```python
from build123d import *

# Parameters (mm, degrees)
SKETCH1_W           = 42
SKETCH1_H           = 62
SKETCH1_R           = 4.15
BOSS_EXTRUDE1_DEPTH = 10
FILLET1_R           = 3
SKETCH2_R           = 2.6
CUT_EXTRUDE1_DEPTH  = 11
SKETCH3_R           = 9.45
CUT_EXTRUDE2_DEPTH  = 10


with BuildPart() as part:
    # Sketch1 → Boss-Extrude1 (new body)
    with BuildSketch(Plane.XY):
        with Locations((21, 31)):
            Rectangle(SKETCH1_W, SKETCH1_H)
        with Locations((21, 42)):
            Circle(SKETCH1_R, mode=Mode.SUBTRACT)
    extrude(amount=BOSS_EXTRUDE1_DEPTH)

    # Fillet1
    fillet1_edges = [part.edges().sort_by_distance(p)[0] for p in [
        (0, 62, 5),
        (42, 62, 5),
    ]]
    fillet(fillet1_edges, radius=FILLET1_R)

    # Sketch2 → Cut-Extrude1 (cut, through all)
    with BuildSketch(Plane.XY.offset(10)):
        with Locations((5, 7.5)):
            Circle(SKETCH2_R)
        with Locations((21, 7.5)):
            Circle(SKETCH2_R)
        with Locations((37, 7.5)):
            Circle(SKETCH2_R)
    extrude(amount=-CUT_EXTRUDE1_DEPTH, mode=Mode.SUBTRACT)

    # Sketch3 → Cut-Extrude2 (cut)
    with BuildSketch(Plane.XY.offset(10)):
        with Locations((21, 42)):
            Circle(SKETCH3_R)
    extrude(amount=-CUT_EXTRUDE2_DEPTH, mode=Mode.SUBTRACT)


solid = part.part
```
Source: CAD feature listing. Evaluate the final solid. Frame: model axes, mm. Round coordinates to 2 decimals unless told otherwise and drop trailing zeros. Loops run counter-clockwise (first coordinate to the right, second up) from the corner with the lowest first, then second, coordinate; pieces in that order, holes last. Notation, with made-up numbers: M 43,66.5 L 53,66.5 A22 cw 53,97.5 Z; hole C -15.75,-28.5 d4. An arc over 180 degrees is marked long. Put each result on its own line as item: value.
(1) Section C-C, the plane x = 21. Return loops of the section in (y, z), and give its area (3 significant figures).
Solutions:
outline: M 0,0 L 4.9,0 L 4.9,10 L 0,10 Z; M 10.1,0 L 32.55,0 L 32.55,10 L 10.1,10 Z; M 51.45,0 L 62,0 L 62,10 L 51.45,10 Z
area: 379 mm²
(2) Ray query, line 1 (Y direction, x = 5, z = 7); line 2 (Y direction, x = 13, z = 7); line 3 (X direction, y = 43, z = 5.5). Return the intervals inside material, ascending. Write a range as [from, to].
Solutions:
line 1: [0, 4.9], [10.1, 62]
line 2: [0, 36.97], [47.03, 62]
line 3: [0, 11.6], [30.4, 42]
(3) Section A-A, the plane y = 42. Return loops of the section in (x, z).
Solutions:
outline: M 0,0 L 11.55,0 L 11.55,10 L 0,10 Z; M 30.45,0 L 42,0 L 42,10 L 30.45,10 Z
(4) Section B-B, the plane x = 37. Return loops of the section in (y, z).
Solutions:
outline: M 0,0 L 4.9,0 L 4.9,10 L 0,10 Z; M 10.1,0 L 62,0 L 62,10 L 10.1,10 Z
(5) First-contact query: pin 1 (6 mm diameter, centred on x = 10, y = 40.5, fed in from -Z). Flat tip, straight axial feed; report the tip coordinate or a pass-through.
Solutions:
pin 1: z = 0
(6) Pull-direction query (X, two-part tool) for faces 1 (the face through (34.937, 5.918, 5.07)), 2 (the face through (41.1, 61.14, 5.07)), 3 (the face through (0.86, 61.1, 5.07)), 4 (the face through (21, 31, 0)); classes: released by +X, released by -X, zero draft, split by the parting line, or undercut.
Solutions:
face 1: undercut
face 2: released by +X
face 3: released by -X
face 4: zero draft
(7) Section D-D, the plane z = 4.25. Return loops of the section in (x, y), and give its area (3 significant figures).
Solutions:
outline: M 0,0 L 42,0 L 42,59 A3 ccw 39,62 L 3,62 A3 ccw 0,59 Z; hole C 5,7.5 d5.2; hole C 21,42 d18.9; hole C 21,7.5 d5.2; hole C 37,7.5 d5.2
area: 2,260 mm²
